Source: CAD feature listing. Evaluate the final solid. Frame: model axes, mm. Give positions to 0.01 mm unless a question says otherwise; leave off trailing zeros. Order: outer loops, then holes, each group sorted by start corner. A loop starts at its lowest first (then second) coordinate and runs counter-clockwise, first axis right, second up. Notation, with made-up numbers: M -14,83 L 15,83 A10 cw 15,94 Z; hole C 51.5,-3 d10. An arc over 180 degrees is marked long. Use CSV: the item, a comma, the result in double quotes. Start each with the question number.
Item 1: First-contact query: pin 1 (1 mm diameter, centred on x = -186.5, y = 3, fed in from +Z). Flat tip, straight axial feed; report the tip coordinate or a pass-through.
Item 2: Section query D-D on x = -150. Return loops of the section in (y, z).
Item 3: Ray query, probe 1 along X at (y, z) = (0.85, 251.5); probe 2 along X at (y, z) = (1.75, -104.5); probe 3 along Z at (x, y) = (243.5, 1.6). Return the intervals inside material, ascending. Write a range as from..to.
Item 4: Section query A-A on x = 0. Return loops of the section in (y, z), and give its area (3 significant figures).
Item 5: Section query C-C on z = 160. Return loops of the section in (x, y), and give its area (3 significant figures).
Item 6: Section query B-B on y = 2.55. Count the separate pieces of the cut face and the enclosed holes in it, and give its area (3 significant figures).
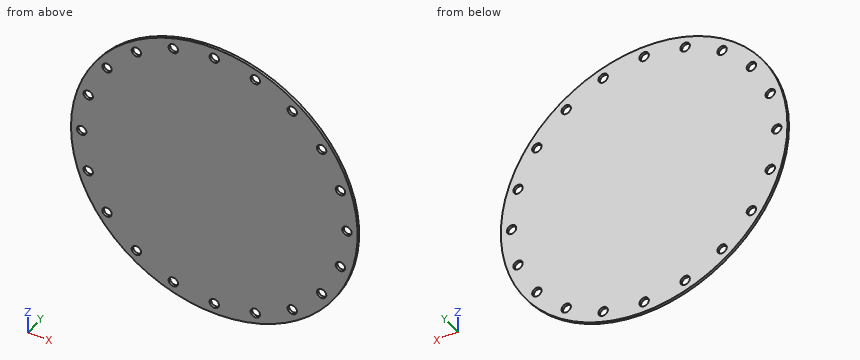
Autodesk Inventor part; units mm, degrees
ref_plane "YZ Plane" through (0, 0, 0) normal (1, 0, 0) x (0, 1, 0)
ref_plane "XZ Plane" through (0, 0, 0) normal (0, 1, 0) x (-1, 0, 0)
ref_plane "XY Plane" through (0, 0, 0) normal (0, 0, 1) x (1, 0, 0)
sketch "Sketch1" plane through (0, 0, 0) normal (0, 1, 0) x (-1, 0, 0)
  circle A0 centre (0, 0) radius 335
  dimension "d0" = 670
extrude "Extrusion1" add sketch "Sketch1" along normal blind 6
sketch "Sketch2" plane through (0, 6, 0) normal (0, 1, 0) x (1, 0, 0)
  circle A0 centre (-310, 0) radius 11
  circle A1 centre (0, 0) radius 310 construction
  dimension "d4" = 620
  dimension "d3" = 22
extrude "Cut1" cut sketch "Sketch2" against normal blind 6
pattern_circular "Circular Pattern1" count 20 over 360 about axis through (0, 0, 0) along (0, 1, 0) of "Cut1"
equation "\"d6\" = Thickness"
equation "\"BendRadius\" = Thickness"
equation "\"BendReliefWidth\" = Thickness"
equation "\"BendReliefDepth\" = 0.5 * Thickness"
equation "\"CornerReliefSize\" = 4 * Thickness"
equation "\"MinimumRemnant\" = 2 * Thickness"
equation "\"TransitionRadius\" = BendRadius"
equation "\"JacobiRadiusSize\" = BendRadius"
equation "\"GapSize\" = Thickness"
equation "\"d5\" = Thickness"
properties part number "PNS-721 charging hatch D1200"
Verdict:
1,pin 1,"z = 278.62"
2,outline,"M 0,-299.54 L 6,-299.54 L 6,299.54 L 0,299.54 Z"
3,probe 1,"-221.3..-193.19, -171.24..171.24, 193.19..221.3"
3,probe 2,"-318.28..-301.55, -288.1..288.1, 301.55..318.28"
3,probe 3,"-230.07..-190.45, -173.98..173.98, 190.45..230.07"
4,outline,"M 0,-335 L 6,-335 L 6,-321 L 0,-321 Z; M 0,-299 L 6,-299 L 6,299 L 0,299 Z; M 0,321 L 6,321 L 6,335 L 0,335 Z"
4,area,"3,760 mm2"
5,outline,"M -294.32,0 L 294.32,0 L 294.32,6 L -294.32,6 Z"
5,area,"3,530 mm2"
6,separate pieces,"1"
6,enclosed holes,"20"
6,area,"345,000 mm2"
